Design review of the part shown in the three views and the two pictorial views. Dimensions are in mm from the part's minimum x, y and z. A direction names the side the tool comes from. Coordinates: 2 decimals unless noted, no trailing zeros. Write each loop counter-clockwise with the first axis right and the second up, starting at its lowest first coordinate (ties: lowest second). Pieces come first, ordered by that corner, then holes. Notation, with made-up numbers: (-18.5, -13) -> (-8.5, -13) arc R10 ccw to (-8.5, -6) -> close; hole circle Ø3 at (-39, 10.25). An arc over 180 degrees is marked (long way). Answer in a Markdown table with one row per item. Add a question column.
Item 1: Take a section at D-D, the plane x = 1.25. Write out the cut boundary in (y, z), and give its area (3 significant figures).
Item 2: Take a section at B-B, the plane y = 5.5. Write out the cut boundary in (x, z) (1 decimal), and give its area (3 significant figures).
Item 3: For the marked faces 1 and 2, list the 3-axis set-ups (+Z, -Z, +X, -X, +Y, -Y) from which the entire face can be reached by the end or side of a thin tool; tool diameter is ignored.
Item 4: Clearance check with a flat-ended pin moving along its axis: P1, Ø0.6, axis at x = 3.5, z = 3.5, coming from the +Y side. State where the tip first meets the part, or that it passes through.
Item 5: To check wall thickness, follow line 1 (Y direction, x = 2.75, z = 3.1) (1 decimal); line 2 (Z direction, x = 1.75, y = 4.25); line 3 (X direction, y = 5.75, z = 4.2). State the ranges of each line that lie inside material, in increasing order.
Item 6: Take a section at C-C, the plane z = 3.35. Write out the cut boundary in (x, y) (1 decimal), and give its area (3 significant figures).
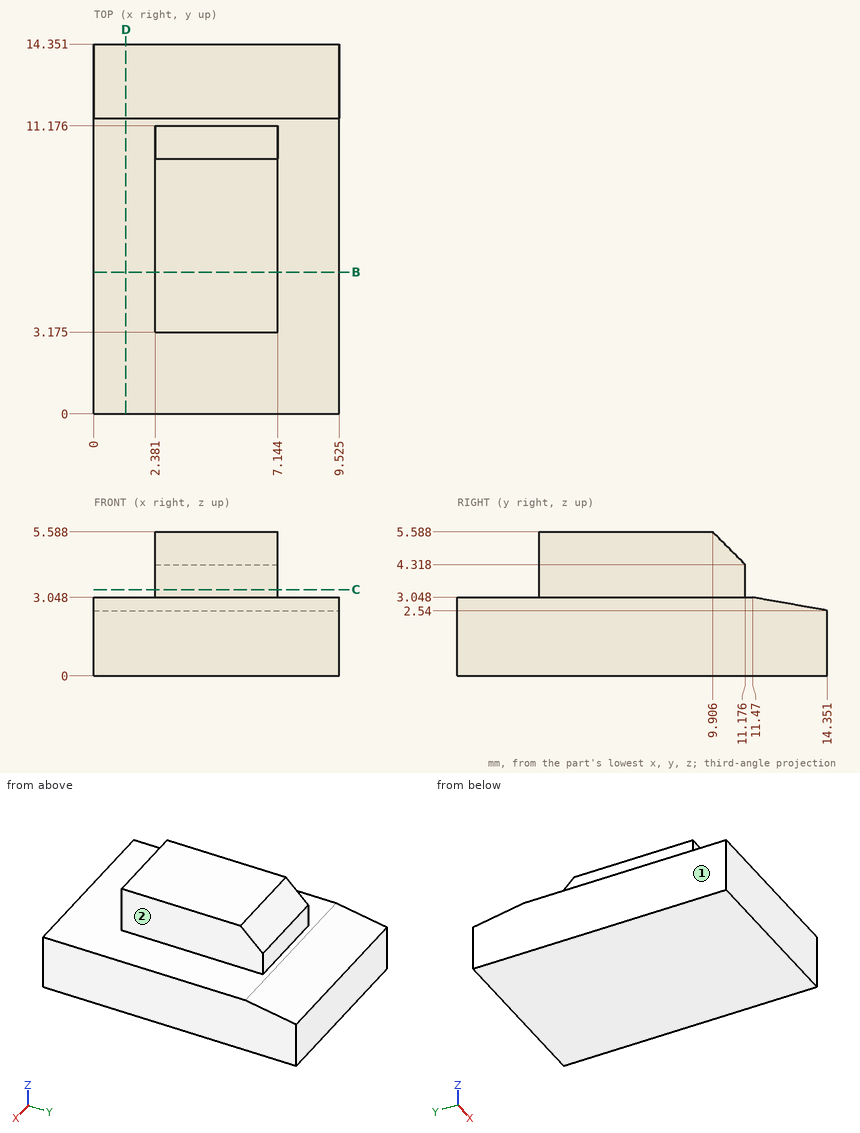
Answers:
| question | item | result |
|---|---|---|
| 1 | outline | (0, 0) -> (14.35, 0) -> (14.35, 2.54) -> (11.47, 3.05) -> (0, 3.05) -> close |
| 1 | area | 43.0 mm^2 |
| 2 | outline | (0, 0) -> (9.5, 0) -> (9.5, 3) -> (7.1, 3) -> (7.1, 5.6) -> (2.4, 5.6) -> (2.4, 3) -> (0, 3) -> close |
| 2 | area | 41.1 mm^2 |
| 3 | face 1 | +Z, -Z, -X, +Y, -Y |
| 3 | face 2 | +Z, +X, +Y, -Y |
| 4 | P1 | stops at y = 11.18 |
| 5 | line 1 | y = 3.2 to 11.2 |
| 5 | line 2 | z = 0 to 3.05 |
| 5 | line 3 | x = 2.38 to 7.14 |
| 6 | outline | (2.4, 3.2) -> (7.1, 3.2) -> (7.1, 11.2) -> (2.4, 11.2) -> close |
| 6 | area | 38.1 mm^2 |
